The listing builds one solid part. Answer for the finished solid, in the listing's coordinates (mm). Face numbers are marked on the shaded views. Round coordinates to 2 decimals unless told otherwise and drop trailing zeros. Put each result on its own line as item: value. Start each with the question number.
1. The mould has two halves that part along X. Classify the marked faces 1 and 2: +X half, -X half, draft (parallel to the pull), parting line (faces both ways), or undercut.
2. Consider line 1 (Y direction, x = 0, z = 27); line 2 (X direction, y = 0, z = 5); line 3 (Y direction, x = 0, z = 9). Determine where each line is inside the solid, lowest interval first.
3. Each of these flat-tipped pins is pushed along its axis until it touches: pin 1 Ø1.3 at (x, y) = (0.5, -1) entering from -Z (3 decimals); pin 2 Ø1.5 at (x, y) = (-17.5, 2.5) entering from -Z; pin 3 Ø5 at (x, y) = (0, 0) entering from +Z (3 decimals); pin 4 Ø1 at (x, y) = (17.5, 15.5) entering from -Z. Where does it stop, or does it pass through?
from build123d import *

# Parameters (mm, degrees)
F2_R     = 4.7625
F3_DEPTH = 9.525
F4_R     = 2.2225
F5_DEPTH = 20.955


with BuildPart() as f1:
    # F0 (on Front) → F1 (revolve)
    with BuildSketch(Plane.XZ):
        with BuildLine():
            Line((0, 31.75), (0, 0))
            add(Edge.make_bspline(
                [(0, 0), (11.3912708933, 5.2234637309), (31.6529425674, 13.3350349717), (15.0865243452, 22.9511441647), (6.35, 25.4)],
                knots=[0, 0, 0, 0, 0.5389896465, 1, 1, 1, 1], degree=3))
            Line((6.35, 25.4), (6.35, 31.75))
            Line((6.35, 31.75), (0, 31.75))
        make_face()
    revolve(axis=Axis((0, 0, 15.875), (0, 0, -1)))

    # F2 (on face) → F3 (cut)
    with BuildSketch(Plane.XY.offset(31.75)):
        Circle(F2_R)
    extrude(amount=-F3_DEPTH, mode=Mode.SUBTRACT)

    # F4 (on Top) → F5 (cut)
    with BuildSketch(Plane.XY):
        Circle(F4_R)
    extrude(amount=F5_DEPTH, mode=Mode.SUBTRACT)


solid = f1.part
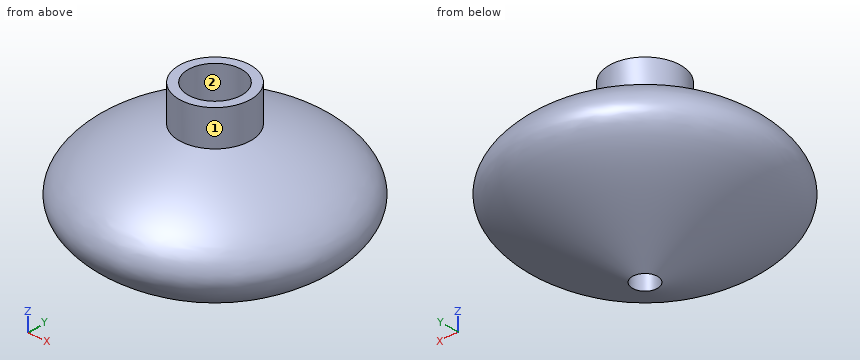
Resolved:
1. face 1: parting line
1. face 2: undercut
2. line 1: -6.35 to -4.76, 4.76 to 6.35
2. line 2: -10.88 to -2.22, 2.22 to 10.88
2. line 3: -18.15 to -2.22, 2.22 to 18.15
3. pin 1: z = 20.955
3. pin 2: z = 8.22
3. pin 3: z = 22.225
3. pin 4: through
